Build history of the part. All positions in model axes, mm. A direction names the side the tool comes from. Give positions to 0.01 mm unless a question says otherwise; leave off trailing zeros. Loops run counter-clockwise (first coordinate to the right, second up) from the corner with the lowest first, then second, coordinate; pieces in that order, holes last. Notation, with made-up numbers: (-10, 26.5) - (45, 26.5) arc R12 ccw to (45, 35.5) - close; hole circle Ø4 at (68.5, 73). An arc over 180 degrees is marked (long way). Return JSON: item names as keys, results as strings. Group by question number.
1) Drill centre lines: probe 1 along Y at (x, z) = (-1.35, 0) (3 decimals); probe 2 along X at (y, z) = (27, 4); probe 3 along Z at (x, y) = (-2.05, 26). Where is each one in solid material? Low to high. Write a range as from..to.
2) Slice it at A-A (y = 23). List the corners of the cut face in (x, z) (3 decimals).
3) Drop flat-ended pins along their axis: pin 1 (0.5 mm diameter, centred on x = -2.5, z = -10.5, fed in from -Y); pin 2 (0.5 mm diameter, centred on x = -3.5, z = 10.5, fed in from +Y); pin 3 (1.2 mm diameter, centred on x = -2.5, y = -3, fed in from -Z). Give the stop position or say it passes through.
4) Slice it at B-B (x = -1.7). List the corners of the cut face in (y, z) (3 decimals), and give its area (3 significant figures).
5) Slice it at D-D (z = -6.5). List the corners of the cut face in (x, y).
6) Slice it at C-C (z = 0). List the corners of the cut face in (x, y) (3 decimals), and give its area (3 significant figures).
7) 3-axis set-ups, long thin cutter, end or side, ignore diameter. For faces 1 (the face through (-3, -2, -10)), 2 (the face through (-1, 40, 0)), 3 (the face through (-2.5, 30, 10.5)), 4 (the face through (-2.5, 0, 10.5)): which of +Z, -Z, +X, -X, +Y, -Y reach the whole face in a straight line?
8) Mould opens along Y. For faces 5 (the face through (-3.732, 19.852, -0.223)), 6 (the face through (-1.23, 34.61, 0.61)), 7 (the face through (-2, 15, -12)), 8 (the face through (-1.232, 31.413, 7.186)) say: released by +Y, released by -Y, zero draft, split by the parting line, or undercut.
```python
from build123d import *

# Parameters (mm, degrees)
SKETCH1_R                = 10
SKETCH1_R_2              = 4.5
SKETCH1_R_3              = 1.275
BOSS_EXTRUDE1_DEPTH      = 2.5
BOSS_EXTRUDE3_DEPTH      = 5
SKETCH2_W                = 5
SKETCH2_H                = 20
BOSS_EXTRUDE4_DEPTH      = 5
BOSS_EXTRUDE5_REACH      = 43.533
SKETCH3_W                = 2
SKETCH3_H                = 30
CHAMFER1_SIZE            = 1
CHAMFER2_SIZE            = 1
OFFSET_FOR_3D_PRINT_BY   = 0.15
OFFSET_FOR_3D_PRINT_2_BY = 0.15
OFFSET_FOR_3D_PRINT_3_BY = 0.15
OFFSET_FOR_3D_PRINT_4_BY = 0.15
OFFSET_FOR_3D_PRINT_5_BY = 0.15
OFFSET_FOR_3D_PRINT_6_BY = 0.15


with BuildPart() as part:
    # Sketch1 → Boss-Extrude1 (new body)
    with BuildSketch(Plane(origin=(0, 0, 0), x_dir=(0, 0, -1), z_dir=(1, 0, 0))):
        with Locations((0, 30)):
            Circle(SKETCH1_R)
        with Locations((0, 30)):
            Circle(SKETCH1_R_2, mode=Mode.SUBTRACT)
        with Locations((7, 30)):
            Circle(SKETCH1_R_3, mode=Mode.SUBTRACT)
        with Locations((0, 23)):
            Circle(SKETCH1_R_3, mode=Mode.SUBTRACT)
        with Locations((-7, 30)):
            Circle(SKETCH1_R_3, mode=Mode.SUBTRACT)
        with Locations((0, 37)):
            Circle(SKETCH1_R_3, mode=Mode.SUBTRACT)
    extrude(amount=-BOSS_EXTRUDE1_DEPTH)

    # Sketch1<6> → Boss-Extrude3 (add)
    with BuildSketch(Plane(origin=(0, 0, 0), x_dir=(0, 0, -1), z_dir=(1, 0, 0))):
        with BuildLine():
            ThreePointArc((10, 30), (0, 20), (-10, 30))
            Line((-10, 30), (-10, 0))
            Line((-10, 0), (10, 0))
            Line((10, 0), (10, 30))
        make_face()
    extrude(amount=-BOSS_EXTRUDE3_DEPTH)


with BuildPart() as body_2:
    # Sketch2 → Boss-Extrude4 (new body)
    with BuildSketch(Plane.XZ):
        with Locations((-2.5, 0)):
            Rectangle(SKETCH2_W, SKETCH2_H)
    extrude(amount=BOSS_EXTRUDE4_DEPTH)


with BuildPart() as part_1:
    add(part.part)

    # Combine2: union body 2
    add(body_2.part)

    # Boss-Extrude5: up to this face of the body (flat: up to its plane)
    boss_extrude5_end = Plane(part_1.part.faces().sort_by_distance((-5, 8.664765534, 0))[0])
    # Sketch3 → Boss-Extrude5 (add, up to the picked face)
    with BuildSketch(Plane(origin=(0, 0, 0), x_dir=(0, 0, -1), z_dir=(1, 0, 0)), mode=Mode.PRIVATE) as boss_extrude5_sk1:
        with Locations((11, 15)):
            Rectangle(SKETCH3_W, SKETCH3_H)
    boss_extrude5_tool1 = split(extrude(boss_extrude5_sk1.sketch, amount=-BOSS_EXTRUDE5_REACH, mode=Mode.PRIVATE), bisect_by=boss_extrude5_end, keep=Keep.BOTH, mode=Mode.PRIVATE)
    # Sketch3 → Boss-Extrude5 (add, up to the picked face)
    with BuildSketch(Plane(origin=(0, 0, 0), x_dir=(0, 0, -1), z_dir=(1, 0, 0)), mode=Mode.PRIVATE) as boss_extrude5_sk2:
        with Locations((-11, 15)):
            Rectangle(SKETCH3_W, SKETCH3_H)
    boss_extrude5_tool2 = split(extrude(boss_extrude5_sk2.sketch, amount=-BOSS_EXTRUDE5_REACH, mode=Mode.PRIVATE), bisect_by=boss_extrude5_end, keep=Keep.BOTH, mode=Mode.PRIVATE)
    add(boss_extrude5_tool1.solids().sort_by(Axis((0, 15, -11), (-1, 0, 0)))[0])
    add(boss_extrude5_tool2.solids().sort_by(Axis((0, 15, 11), (-1, 0, 0)))[0])

    # Chamfer1
    chamfer1_edges = [part_1.edges().sort_by_distance(p)[0] for p in [
        (-2.5, 0, -12),
        (-2.5, 30, -12),
        (-2.5, 30, 12),
        (-2.5, 0, 12),
    ]]
    chamfer(chamfer1_edges, length=CHAMFER1_SIZE)

    # Chamfer2
    chamfer2_edges = [part_1.edges().sort_by_distance(p)[0] for p in [
        (-2.5, -5, -10),
        (-2.5, -5, 10),
    ]]
    chamfer(chamfer2_edges, length=CHAMFER2_SIZE)

    # Offset for 3D print: a curved face moved inward by 0.15
    add(Solid.thicken(part_1.faces().sort_by_distance((-3.75, 20, 0))[0], -OFFSET_FOR_3D_PRINT_BY), mode=Mode.SUBTRACT)

    # Offset for 3D print 2: a curved face moved inward by 0.15
    add(Solid.thicken(part_1.faces().sort_by_distance((-1.25, 37, 1.275))[0], -OFFSET_FOR_3D_PRINT_2_BY), mode=Mode.SUBTRACT)

    # Offset for 3D print 3: a curved face moved inward by 0.15
    add(Solid.thicken(part_1.faces().sort_by_distance((-1.25, 23, 1.275))[0], -OFFSET_FOR_3D_PRINT_3_BY), mode=Mode.SUBTRACT)

    # Offset for 3D print 4: a curved face moved inward by 0.15
    add(Solid.thicken(part_1.faces().sort_by_distance((-1.25, 30, -5.725))[0], -OFFSET_FOR_3D_PRINT_4_BY), mode=Mode.SUBTRACT)

    # Offset for 3D print 5: a curved face moved inward by 0.15
    add(Solid.thicken(part_1.faces().sort_by_distance((-1.25, 30, 8.275))[0], -OFFSET_FOR_3D_PRINT_5_BY), mode=Mode.SUBTRACT)

    # Offset for 3D print 6: a curved face moved inward by 0.15
    add(Solid.thicken(part_1.faces().sort_by_distance((-1.25, 30, 4.5))[0], -OFFSET_FOR_3D_PRINT_6_BY), mode=Mode.SUBTRACT)


solid = part_1.part
```
Results:
{
 "1": {"probe 1": "-5..21.575, 24.425..25.35, 34.65..35.575, 38.425..40", "probe 2": "-2.5..0", "probe 3": "-12..-2.37, 2.37..12"},
 "2": {"outline": "(-5, -12) - (0, -12) - (0, -1.425) - (-2.5, -1.425) - (-2.5, -7.35) - (-5, -7.35) - close; (-5, 7.35) - (-2.5, 7.35) - (-2.5, 1.425) - (0, 1.425) - (0, 12) - (-5, 12) - close"},
 "3": {"pin 1": "y = 0", "pin 2": "y = 30", "pin 3": "z = -10"},
 "4": {"outline": "(-5, -9) - (-4, -10) - (0, -10) - (0, -11) - (1, -12) - (29, -12) - (30, -11) - (30, -10) arc R10 ccw to (30, 10) - (30, 11) - (29, 12) - (1, 12) - (0, 11) - (0, 10) - (-4, 10) - (-5, 9) - close; hole circle Ø2.85 at (23, 0); hole circle Ø9.3 at (30, 0); hole circle Ø2.85 at (30, -7); hole circle Ø2.85 at (30, 7); hole circle Ø2.85 at (37, 0)", "area": "881 mm2"},
 "5": {"outline": "(-5, -5) - (0, -5) - (0, 28.67) - (-2.5, 28.67) - (-2.5, 22.2) - (-5, 22.2) - close; (-2.5, 31.33) - (0, 31.33) - (0, 37.6) - (-2.5, 37.6) - close"},
 "6": {"outline": "(-5, -5) - (0, -5) - (0, 21.575) - (-2.5, 21.575) - (-2.5, 19.85) - (-5, 19.85) - close; (-2.5, 24.425) - (0, 24.425) - (0, 25.35) - (-2.5, 25.35) - close; (-2.5, 34.65) - (0, 34.65) - (0, 35.575) - (-2.5, 35.575) - close; (-2.5, 38.425) - (0, 38.425) - (0, 40) - (-2.5, 40) - close", "area": "137 mm2"},
 "7": {"face 1": "-Z, +X, -X, -Y", "face 2": "+X, -X, +Y", "face 3": "+Z, +X, -X, +Y", "face 4": "+Z, +X, -X, -Y"},
 "8": {"face 5": "released by +Y", "face 6": "undercut", "face 7": "zero draft", "face 8": "undercut"}
}
